Geometry check sheet. Reference: the model listing, model coordinates, mm. A direction names the side the tool comes from. Coordinates: 2 decimals unless noted, no trailing zeros. Order: outer loops, then holes, each group sorted by start corner. A loop starts at its lowest first (then second) coordinate and runs counter-clockwise, first axis right, second up. Notation, with made-up numbers: (12, 79) -> (68, 79) arc R8 cw to (68, 84) -> close; hole circle Ø5 at (8, 26.5). An arc over 180 degrees is marked (long way). Answer in a Markdown table with one row per item. Add a question column.
Autodesk Fusion 360 part; units mm, degrees
sketch "Esquisse1" plane through (0, 0, 0) normal (0, 0, 1) x (1, 0, 0)
  line L0 (-40, 10) -> (40, 10)
  line L1 (40, 10) -> (40, -10)
  line L2 (40, -10) -> (-40, -10)
  line L3 (-40, -10) -> (-40, 10)
extrude "Extrusion1" add sketch "Esquisse1" along normal blind 10
sketch "Esquisse2" plane through (0, 0, 10) normal (0, 0, 1) x (-1, 0, 0)
  line L0 (40, 10) -> (-40, 10)
  line L1 (-40, 10) -> (-40, -10)
  line L2 (-40, -10) -> (40, -10)
  line L3 (40, -10) -> (40, 10)
  line L4 (15, -10) -> (-15, -10)
  line L5 (-15, -10) -> (-15, 10)
  line L6 (-15, 10) -> (15, 10)
  line L7 (15, 10) -> (15, -10)
  circle A0 centre (-31.183, 0) radius 1.625
  circle A1 centre (31.183, 0) radius 1.625
  dimension "d7" = 3.25
  dimension "d8" = 3.25
extrude "Extrusion2" cut sketch "Esquisse2" against normal blind 10 contours A1
extrude "Extrusion3" cut sketch "Esquisse2" against normal blind 10 contours A0
extrude "Extrusion4" add sketch "Esquisse2" along normal blind 30 contours L0 L2 L4 L5 L6 L7
sketch "Esquisse3" plane through (0, -10, 0) normal (0, -1, 0) x (1, 0, 0)
  line L0 (-40, 0) -> (40, 0)
  line L1 (40, 0) -> (40, 10)
  line L2 (40, 10) -> (15, 10)
  line L3 (15, 10) -> (15, 40)
  line L4 (15, 40) -> (-15, 40)
  line L5 (-15, 40) -> (-15, 10)
  line L6 (-15, 10) -> (-40, 10)
  line L7 (-40, 10) -> (-40, 0)
  circle A0 centre (0, 25) radius 6.5
  circle A1 centre (0, 25) radius 8
  dimension "d15" = 13
  dimension "d16" = 16
extrude "Extrusion5" cut sketch "Esquisse3" against normal blind 20 contours A0
extrude "Extrusion6" cut sketch "Esquisse3" against normal blind 5.1 contours A1
sketch "Esquisse4" plane through (0, 0, 40) normal (0, 0, 1) x (-1, 0, 0)
  line L0 (15, 10) -> (-15, 10)
  line L1 (-15, 10) -> (-15, -10)
  line L2 (-15, -10) -> (15, -10)
  line L3 (15, -10) -> (15, 10)
  line L4 (15, 10) -> (10, 10)
  line L5 (10, 10) -> (10, -5)
  line L6 (10, -5) -> (15, -5)
  line L7 (15, -5) -> (15, 10)
  line L8 (-15, 10) -> (-10, 10)
  line L9 (-10, 10) -> (-10, -5)
  line L10 (-10, -5) -> (-15, -5)
  line L11 (-15, -5) -> (-15, 10)
extrude "Extrusion7" add sketch "Esquisse4" along normal blind 10 contours L0 L3 L4 L5 L6 L7 | L0 L1 L8 L9 L10 L11
sketch "Esquisse5" plane through (0, 0, 50) normal (0, 0, 1) x (-1, 0, 0)
  line L0 (15, -5) -> (15, 10)
  line L1 (15, 10) -> (10, 10)
  line L2 (10, 10) -> (10, -5)
  line L3 (10, -5) -> (15, -5)
  line L4 (15, -5) -> (-15, -5)
  line L5 (-15, -5) -> (-15, 10)
  line L6 (-15, 10) -> (15, 10)
  line L7 (15, 10) -> (15, -5)
extrude "Extrusion8" add sketch "Esquisse5" along normal blind 5
extrude "Extrusion9" cut 1 faces at (-3.3333, 0, 55) along direction (0, 0, -1) blind 5
extrude "Extrusion10" cut 2 faces at (-13.3333, 0, 50) (13.3333, -5, 50) along direction (0, 0, -1) blind 10
(1) Go/stop test with flat-tipped pins: P1, Ø10, axis at x = -33, y = -3.5, coming from the +Z side; P2, Ø11.5, axis at x = 0, z = 25, coming from the -Y side; P3, Ø10, axis at y = 1.5, z = 18, coming from the +X side. Record where each tip stops, or that it passes through.
(2) Scan lines: line 1 along X through (y, z) = (0, 2); line 2 along Z through (x, y) = (-36, 8.25); line 3 along X through (y, z) = (-2.5, 28.5). Record each from-to range of solid material in increasing order.
(3) Mould release check, pull along Z, two halves, no side actions. Record for faces 5 (the face through (-0.846, 2.446, 31.445)), 6 (the face through (-15, 0, 25)), 7 (the face through (0, -4.9, 32)), 8 (the face through (27, 0, 10)): +Z half, -Z half, draft (parallel to the pull), parting line (faces both ways), or undercut.
(4) Cross-section at B-B (z = 25). Enter the section's corners in (x, y), plus the area to 3 significant figures.
(5) Cross-section at D-D (x = 0). Enter the section's corners in (y, z), plus the area to 3 significant figures.
(6) Cross-section at A-A (y = 0). Enter the section's corners in (x, z), plus the area to 3 significant figures.
(7) Cross-section at C-C (y = 5.5). Enter the section's corners in (x, z).
(8) Access from +Z, -Z, +X, -X, +Y, -Y to the whole of each face (thin tool, end or side, straight path). Record for faces 1 (the face through (-28, 0, 10)), 2 (the face through (-1.041, -7.486, 32.932)), 3 (the face through (15, 0, 25)), 4 (the face through (1, -10, 15)).
Checks:
| question | item | result |
|---|---|---|
| 1 | P1 | z = 10 |
| 1 | P2 | through |
| 1 | P3 | x = 15 |
| 2 | line 1 | -40 to -32.81, -29.56 to 29.56, 32.81 to 40 |
| 2 | line 2 | 0 to 10 |
| 2 | line 3 | -15 to -5.48, 5.48 to 15 |
| 3 | face 5 | undercut |
| 3 | face 6 | draft |
| 3 | face 7 | undercut |
| 3 | face 8 | +Z half |
| 4 | outline | (-15, -10) -> (-8, -10) -> (-8, -4.9) -> (-6.5, -4.9) -> (-6.5, 10) -> (-15, 10) -> close; (6.5, -4.9) -> (8, -4.9) -> (8, -10) -> (15, -10) -> (15, 10) -> (6.5, 10) -> close |
| 4 | area | 325 mm² |
| 5 | outline | (-10, 0) -> (10, 0) -> (10, 18.5) -> (-4.9, 18.5) -> (-4.9, 17) -> (-10, 17) -> close; (-10, 33) -> (-4.9, 33) -> (-4.9, 31.5) -> (10, 31.5) -> (10, 40) -> (-10, 40) -> close |
| 5 | area | 525 mm² |
| 6 | outline | (-40, 0) -> (-32.81, 0) -> (-32.81, 10) -> (-40, 10) -> close; (-29.56, 0) -> (29.56, 0) -> (29.56, 10) -> (15, 10) -> (15, 40) -> (-15, 40) -> (-15, 10) -> (-29.56, 10) -> close; (32.81, 0) -> (40, 0) -> (40, 10) -> (32.81, 10) -> close; hole circle Ø13 at (0, 25) |
| 6 | area | 1,500 mm² |
| 7 | outline | (-40, 0) -> (40, 0) -> (40, 10) -> (15, 10) -> (15, 40) -> (-15, 40) -> (-15, 10) -> (-40, 10) -> close; hole circle Ø13 at (0, 25) |
| 8 | face 1 | +Z, -X, +Y, -Y |
| 8 | face 2 | -Y |
| 8 | face 3 | +Z, +X, +Y, -Y |
| 8 | face 4 | +Z, -Z, +X, -X, -Y |
